The figure shows three views and two pictorial views of one solid part (mm, origin at its lowest corner). Answer the questions. A direction names the side the tool comes from. Coordinates: 2 decimals unless noted, no trailing zeros. Order: outer loops, then holes, each group sorted by start corner. A loop starts at its lowest first (then second) coordinate and runs counter-clockwise, first axis right, second up. Notation, with made-up numbers: (86.5, 74.5) -> (95.5, 74.5) arc R11 ccw to (95.5, 82.5) -> close; hole circle Ø4 at (-26.75, 19.25). An arc over 180 degrees is marked (long way). Return JSON: item names as keys, results as strings.
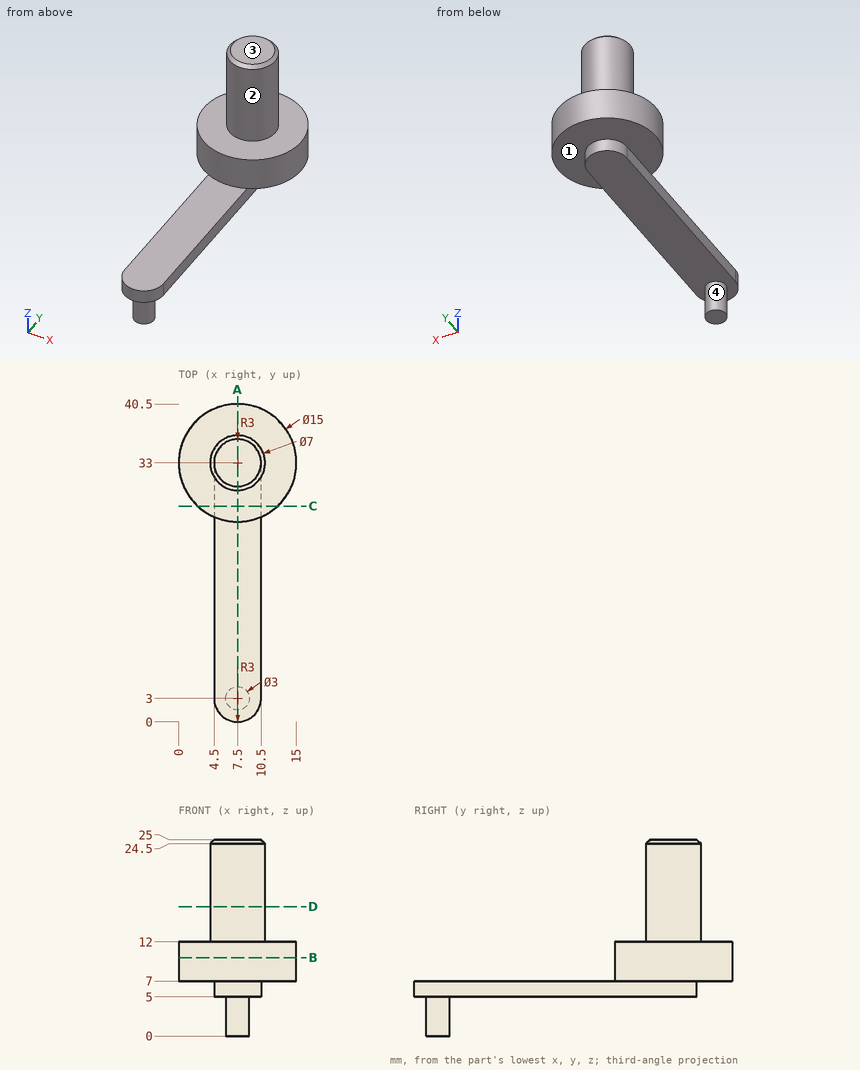
Item 1: Flat-ended cylindrical pins translate along their axes: pin 1 (6 mm diameter, centred on x = 6.5, y = 34.5, fed in from -Z); pin 2 (0.6 mm diameter, centred on y = 12, z = 6.5, fed in from +X); pin 3 (1 mm diameter, centred on x = 12, z = 6, fed in from -Y); pin 4 (1 mm diameter, centred on x = 4.5, z = 14, fed in from +Y). Find the tip coordinate at first contact, or state that the pin passes through.
Answer list:
{"pin 1": "z = 5", "pin 2": "x = 10.5", "pin 3": "through", "pin 4": "y = 35.45"}
Item 2: The part is cut by section D-D on z = 16.5. Determine the outline of the cut face in (x, y).
Answer list:
{"outline": "circle Ø7 at (7.5, 33)"}
Item 3: The part is cut by section B-B on z = 10. Determine the outline of the cut face in (x, y).
Answer list:
{"outline": "circle Ø15 at (7.5, 33)"}
Item 4: Find the intervals of material crossed by probe 1 along Z at (x, y) = (8.5, 2.5); probe 2 along Z at (x, y) = (12.25, 31.5); probe 3 along X at (y, z) = (14, 6.25), in increasing order.
Answer list:
{"probe 1": "0 to 7", "probe 2": "7 to 12", "probe 3": "4.5 to 10.5"}
Item 5: The part is cut by section C-C on y = 27.5. Determine the outline of the cut face in (x, z).
Answer list:
{"outline": "(2.4, 7) -> (4.5, 7) -> (4.5, 5) -> (10.5, 5) -> (10.5, 7) -> (12.6, 7) -> (12.6, 12) -> (2.4, 12) -> close"}
Item 6: The part is cut by section A-A on x = 7.5. Determine the outline of the cut face in (y, z), plus the area to 3 significant figures.
Answer list:
{"outline": "(0, 5) -> (1.5, 5) -> (1.5, 0) -> (4.5, 0) -> (4.5, 5) -> (36, 5) -> (36, 7) -> (40.5, 7) -> (40.5, 12) -> (36.5, 12) -> (36.5, 24.5) -> (36, 25) -> (30, 25) -> (29.5, 24.5) -> (29.5, 12) -> (25.5, 12) -> (25.5, 7) -> (0, 7) -> close", "area": "253 mm2"}
Item 7: Which of the six approach directions +Z, -Z, +X, -X, +Y, -Y give full straight-line access (tool end or side, diameter ignored) to the marked faces 1, 2, 3 and 4?
Answer list:
{"face 1": "-Z, +Y", "face 2": "+Z", "face 3": "+Z, +X, -X, +Y, -Y", "face 4": "-Z"}
